Source: CAD feature listing. Evaluate the final solid. Frame: model axes, mm. A direction names the side the tool comes from. Give positions to 0.01 mm unless a question says otherwise; leave off trailing zeros. Loops run counter-clockwise (first coordinate to the right, second up) from the corner with the lowest first, then second, coordinate; pieces in that order, holes last. Notation, with made-up numbers: (66.5, 60) -> (80.5, 60) arc R22 cw to (80.5, 76) -> close; hole circle Ø1 at (-15, 83). An arc over 180 degrees is marked (long way). Return JSON: item names as keys, results as strings. Group by question number.
(1) Cut plane A-A on z = 505.8. Return loops of the section in (x, y), then the cut area to 3 significant figures.
(2) Pin query (flat end, axial travel): pin 1 (10 mm diameter, centred on x = 21, y = 34.5, fed in from -Z); pin 2 (2 mm diameter, centred on x = 21, z = 281, fed in from +Y); pin 3 (4 mm diameter, centred on x = 21.5, z = 377, fed in from +Y). Return the tip coordinate at first contact, or that it passes through.
(3) Access query for faces 5 (the face through (3, 25, 264)), 6 (the face through (0, 25, 264)). Directions: +Z, -Z, +X, -X, +Y, -Y. A direction counts if a zero-diameter tool reaches every point of the face in a straight line with its end or side. Return the directions, or none.
(4) Cut plane B-B on x = 14.75. Return loops of the section in (y, z).
(5) Cut plane D-D on z = 257.5. Return loops of the section in (x, y), then the cut area to 3 significant figures.
(6) Ray query, line 1 (X direction, y = 6.5, z = 142); line 2 (Y direction, x = 11, z = 37.5); line 3 (Z direction, x = 23.3, y = 25) (3 decimals). Return the intervals inside material, ascending. Write a range as from..to.
(7) Cut plane C-C on y = 25. Return loops of the section in (x, z) (3 decimals).
(8) Draft query along Z for faces 1 (the face through (22.708, 25.117, 16.944)), 2 (the face through (23.482, 23.698, 515.715)), 3 (the face through (12, 0, 262)), 4 (the face through (2, 23, 530.8)). Return one class per face: released by +Z, released by -Z, zero draft, split by the parting line, or undercut.
```python
from build123d import *

# Parameters (mm, degrees)
BOSS_EXTRUDE1_DEPTH = 530.8
SKETCH2_R           = 10
CUT_EXTRUDE1_DEPTH  = 534.733736359
SKETCH2_6_R         = 10
CUT_EXTRUDE2_DEPTH  = 534.733736359


with BuildPart() as part:
    # Sketch1 → Boss-Extrude1 (new body)
    with BuildSketch(Plane.XY):
        with BuildLine():
            Line((0, 44), (0, 6))
            ThreePointArc((0, 6), (1.757359313, 1.757359313), (6, 0))
            Line((6, 0), (18.96119643, 0))
            ThreePointArc((18.96119643, 0), (23.203837117, 1.757359313), (24.96119643, 6))
            Line((24.96119643, 6), (24.96119643, 44))
            ThreePointArc((24.96119643, 44), (23.203837117, 48.242640687), (18.96119643, 50))
            Line((18.96119643, 50), (6, 50))
            ThreePointArc((6, 50), (1.757359313, 48.242640687), (0, 44))
        make_face()
        with BuildLine():
            Line((3, 44), (3, 6))
            ThreePointArc((3, 6), (3.878679656, 3.878679656), (6, 3))
            Line((6, 3), (18.96119643, 3))
            ThreePointArc((18.96119643, 3), (21.082516774, 3.878679656), (21.96119643, 6))
            Line((21.96119643, 6), (21.96119643, 44))
            ThreePointArc((21.96119643, 44), (21.082516774, 46.121320344), (18.96119643, 47))
            Line((18.96119643, 47), (6, 47))
            ThreePointArc((6, 47), (3.878679656, 46.121320344), (3, 44))
        make_face(mode=Mode.SUBTRACT)
    extrude(amount=BOSS_EXTRUDE1_DEPTH)

    # Sketch2 → Cut-Extrude1 (cut, through all)
    with BuildSketch(Plane(origin=(24.96119643, 0, 0), x_dir=(0, 0, -1), z_dir=(1, 0, 0))):
        with Locations(Location((-505.8, 25, 0), (0, 0, 90))):
            Circle(SKETCH2_R)
        Polygon((-33.73, 50), (0, 0), (0, 50), align=None)
    extrude(amount=-CUT_EXTRUDE1_DEPTH, mode=Mode.SUBTRACT)

    # Sketch2_6 → Cut-Extrude2 (cut, through all)
    with BuildSketch(Plane(origin=(24.96119643, 0, 0), x_dir=(0, 0, -1), z_dir=(1, 0, 0))):
        with Locations(Location((-135.8, 25, 0), (0, 0, 90))):
            Circle(SKETCH2_6_R)
    extrude(amount=-CUT_EXTRUDE2_DEPTH, mode=Mode.SUBTRACT)


solid = part.part
```
Answers:
{
 "1": {"outline": "(0, 6) arc R6 ccw to (6, 0) -> (18.96, 0) arc R6 ccw to (24.96, 6) -> (24.96, 15) -> (21.96, 15) -> (21.96, 6) arc R3 cw to (18.96, 3) -> (6, 3) arc R3 cw to (3, 6) -> (3, 15) -> (0, 15) -> close; (0, 35) -> (3, 35) -> (3, 44) arc R3 cw to (6, 47) -> (18.96, 47) arc R3 cw to (21.96, 44) -> (21.96, 35) -> (24.96, 35) -> (24.96, 44) arc R6 ccw to (18.96, 50) -> (6, 50) arc R6 ccw to (0, 44) -> close", "area": "271 mm²"},
 "2": {"pin 1": "z = 19.96", "pin 2": "y = 49.91", "pin 3": "y = 49.98"},
 "3": {"face 5": "+Z, -Z", "face 6": "+Z, -Z, -X, +Y, -Y"},
 "4": {"outline": "(0, 0) -> (3, 2.02) -> (3, 530.8) -> (0, 530.8) -> close; (47, 31.71) -> (50, 33.73) -> (50, 530.8) -> (47, 530.8) -> close"},
 "5": {"outline": "(0, 6) arc R6 ccw to (6, 0) -> (18.96, 0) arc R6 ccw to (24.96, 6) -> (24.96, 44) arc R6 ccw to (18.96, 50) -> (6, 50) arc R6 ccw to (0, 44) -> close; hole (3, 6) arc R3 ccw to (6, 3) -> (18.96, 3) arc R3 ccw to (21.96, 6) -> (21.96, 44) arc R3 ccw to (18.96, 47) -> (6, 47) arc R3 ccw to (3, 44) -> close", "area": "391 mm²"},
 "6": {"line 1": "0..3, 21.96..24.96", "line 2": "0..3, 47..50", "line 3": "16.865..125.8, 145.8..495.8, 515.8..530.8"},
 "7": {"outline": "(0, 16.865) -> (3, 16.865) -> (3, 125.8) -> (0, 125.8) -> close; (0, 145.8) -> (3, 145.8) -> (3, 495.8) -> (0, 495.8) -> close; (0, 515.8) -> (3, 515.8) -> (3, 530.8) -> (0, 530.8) -> close; (21.961, 16.865) -> (24.961, 16.865) -> (24.961, 125.8) -> (21.961, 125.8) -> close; (21.961, 145.8) -> (24.961, 145.8) -> (24.961, 495.8) -> (21.961, 495.8) -> close; (21.961, 515.8) -> (24.961, 515.8) -> (24.961, 530.8) -> (21.961, 530.8) -> close"},
 "8": {"face 1": "released by -Z", "face 2": "undercut", "face 3": "zero draft", "face 4": "released by +Z"}
}
